Input: part model. Units: mm. Frame: model coordinates. Face numbers are marked on the shaded views. A direction names the side the tool comes from. Coordinates: 2 decimals unless noted, no trailing zeros. Order: outer loops, then holes, each group sorted by start corner. A loop starts at its lowest first (then second) coordinate and runs counter-clockwise, first axis right, second up.
from build123d import *

# Parameters (mm, degrees)
F0_W     = 50.8
F0_H     = 25.4
F1_DEPTH = 88.9
F3_DEPTH = 76.2
F2_W     = 63.5
F2_H     = 12.7
F4_DEPTH = 25.4
F5_W     = 38.1
F5_H     = 50.8
F6_DEPTH = 110.744


with BuildPart() as f1:
    # F0 (on Top) → F1 (new body)
    with BuildSketch(Plane.XY):
        Polygon((-60.758203, -51.781196), (-9.958203, -51.781196), (-9.958203, -26.381196), (-9.958203, 24.418804), (-9.958203, 49.818804), (-60.758203, 49.818804), align=None)
        with Locations((15.441797, -39.081196)):
            Rectangle(F0_W, F0_H)
        Polygon((40.841797, -26.381196), (40.841797, -51.781196), (91.641797, -51.781196), (91.641797, 49.818804), (40.841797, 49.818804), (40.841797, 24.418804), align=None)
        with Locations((15.441797, 37.118804)):
            Rectangle(F0_W, F0_H)
    extrude(amount=F1_DEPTH)

    # F2 (on face) → F3 (cut)
    with BuildSketch(Plane.XY.offset(88.9)):
        Polygon((-54.408203, 43.468804), (-54.408203, -45.431196), (-16.308203, -45.431196), (-16.308203, -32.731196), (-16.308203, 30.768804), (-16.308203, 43.468804), align=None)
        Polygon((47.191797, -32.731196), (47.191797, -45.431196), (85.291797, -45.431196), (85.291797, 43.468804), (47.191797, 43.468804), (47.191797, 30.768804), align=None)
    extrude(amount=-F3_DEPTH, mode=Mode.SUBTRACT)

    # F2 (on face) → F4 (cut)
    with BuildSketch(Plane.XY.offset(88.9)):
        with Locations((15.441797, -39.081196)):
            Rectangle(F2_W, F2_H)
        with Locations((15.441797, 37.118804)):
            Rectangle(F2_W, F2_H)
    extrude(amount=-F4_DEPTH, mode=Mode.SUBTRACT)

    # F5 (on face) → F6 (cut)
    with BuildSketch(Plane.XZ.offset(51.781196)):
        with Locations((15.441797, 25.4)):
            Rectangle(F5_W, F5_H)
    extrude(amount=-F6_DEPTH, mode=Mode.SUBTRACT)


solid = f1.part
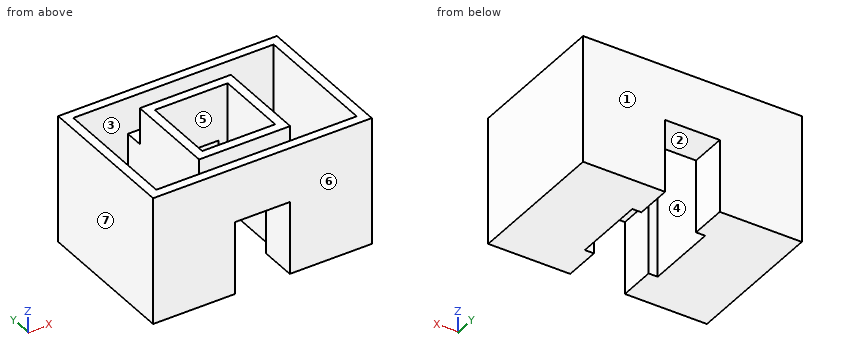
Item 1: Cut plane B-B on y = 19. Return loops of the section in (x, z), then the cut area to 3 significant figures.
Response values:
outline: (-60.76, 0) - (-9.96, 0) - (-9.96, 88.9) - (-16.31, 88.9) - (-16.31, 12.7) - (-54.41, 12.7) - (-54.41, 88.9) - (-60.76, 88.9) - close; (40.84, 0) - (91.64, 0) - (91.64, 88.9) - (85.29, 88.9) - (85.29, 12.7) - (47.19, 12.7) - (47.19, 88.9) - (40.84, 88.9) - close
area: 3,230 mm2
Item 2: Cut plane A-A on z = 72. Return loops of the section in (x, y), then the cut area to 3 significant figures.
Response values:
outline: (-60.76, -51.78) - (91.64, -51.78) - (91.64, 49.82) - (-60.76, 49.82) - close; (-16.31, -32.73) - (47.19, -32.73) - (47.19, 30.77) - (-16.31, 30.77) - close; hole (-54.41, -45.43) - (85.29, -45.43) - (85.29, 43.47) - (-54.41, 43.47) - close; hole (-9.96, -26.38) - (40.84, -26.38) - (40.84, 24.42) - (-9.96, 24.42) - close
area: 4,520 mm2
Item 3: Draft query along Y for the marked faces 5, 6 and 7. Return one class per face: pulls with the +Y half, pulls with the -Y half, needs draft (parallel to the pull), parting line crosses it, or undercut.
Response values:
face 5: undercut
face 6: pulls with the -Y half
face 7: needs draft
Item 4: Cut plane D-D on x = -21. Return loops of the section in (y, z).
Response values:
outline: (-51.78, 0) - (49.82, 0) - (49.82, 88.9) - (43.47, 88.9) - (43.47, 12.7) - (-45.43, 12.7) - (-45.43, 88.9) - (-51.78, 88.9) - close
Item 5: Pin query (flat end, axial travel): pin 1 Ø7.5 at (x, y) = (15, 39) entering from -Z; pin 2 Ø4 at (x, y) = (29, 35) entering from +Z; pin 3 Ø11.5 at (x, y) = (-38.5, -18) entering from +Z. Return the tip coordinate at first contact, or that it passes through.
Response values:
pin 1: stops at z = 50.8
pin 2: stops at z = 63.5
pin 3: stops at z = 12.7
Item 6: Ray query, probe 1 along X at (y, z) = (-38, 52); probe 2 along X at (y, z) = (-20, 74); probe 3 along X at (y, z) = (30.5, 33). Return the intervals inside material, ascending.
Response values:
probe 1: x = -60.76 to -54.41, -16.31 to 47.19, 85.29 to 91.64
probe 2: x = -60.76 to -54.41, -16.31 to -9.96, 40.84 to 47.19, 85.29 to 91.64
probe 3: x = -60.76 to -54.41, -16.31 to -3.61, 34.49 to 47.19, 85.29 to 91.64
Item 7: Access query for the marked faces 1, 2, 3 and 4. Directions: +Z, -Z, +X, -X, +Y, -Y. A direction counts if a zero-diameter tool reaches every point of the face in a straight line with its end or side. Return the directions, or none.
Response values:
face 1: +Z, -Z, +X, -X, +Y
face 2: -Z, +Y, -Y
face 3: +Z
face 4: +Z, -Z
Item 8: Cut plane C-C on x = 24.5. Return loops of the section in (y, z).
Response values:
outline: (-51.78, 50.8) - (-26.38, 50.8) - (-26.38, 88.9) - (-32.73, 88.9) - (-32.73, 63.5) - (-45.43, 63.5) - (-45.43, 88.9) - (-51.78, 88.9) - close; (24.42, 50.8) - (49.82, 50.8) - (49.82, 88.9) - (43.47, 88.9) - (43.47, 63.5) - (30.77, 63.5) - (30.77, 88.9) - (24.42, 88.9) - close
